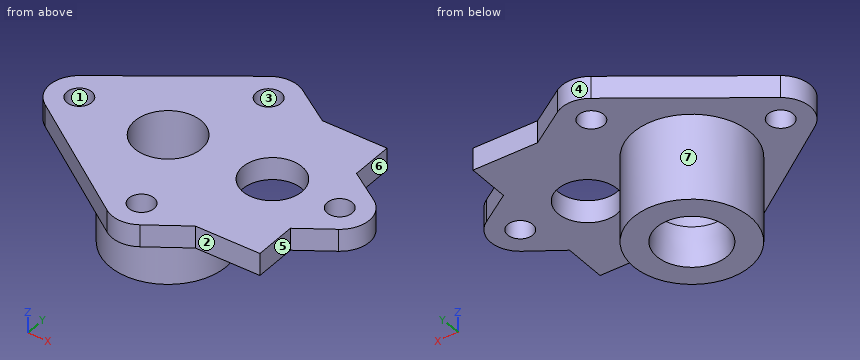
```python
from build123d import *

# Parameters (mm, degrees)
SZKIC1_R                    = 7.9
SZKIC1_R_2                  = 4.75
DODANIE_WYCI_GNI_CIE1_DEPTH = 11.6
DODANIE_WYCI_GNI_CIE2_START = -0.5
SZKIC2_R                    = 4.75
SZKIC2_R_2                  = 4.5
DODANIE_WYCI_GNI_CIE2_DEPTH = 0.5
SFAZOWANIE1_SIZE            = 11.5
SFAZOWANIE1_SIZE_2          = 0.5
SZKIC4_R                    = 4
SZKIC4_R_2                  = 1.7
SZKIC4_R_3                  = 4.5
DODANIE_WYCI_GNI_CIE4_DEPTH = 3
DODANIE_WYCI_GNI_CIE5_DEPTH = 3


with BuildPart() as part:
    # Szkic1 → Dodanie-wyciągnięcie1 (new body)
    with BuildSketch(Plane.XY):
        Circle(SZKIC1_R)
        Circle(SZKIC1_R_2, mode=Mode.SUBTRACT)
    extrude(amount=DODANIE_WYCI_GNI_CIE1_DEPTH)

    # Szkic2 → Dodanie-wyciągnięcie2 (add)
    with BuildSketch(Plane.XY.offset(11.6).offset(DODANIE_WYCI_GNI_CIE2_START)):
        Circle(SZKIC2_R)
        Circle(SZKIC2_R_2, mode=Mode.SUBTRACT)
    extrude(amount=DODANIE_WYCI_GNI_CIE2_DEPTH)

    # Sfazowanie1
    # the kernel refuses this chamfer: 11.5, 0.5 mm, written as the material it adds along each edge
    with BuildSketch(Plane(origin=(0, 0, 11.1), x_dir=(1, 0, 0), z_dir=(0, -1, 0))) as sfazowanie1_piece_1_section:
        Polygon((4.75, -SFAZOWANIE1_SIZE), (4.75 - SFAZOWANIE1_SIZE_2, 0), (4.75, 0), align=None)
    sfazowanie1_piece_1 = revolve(axis=Axis((0, 0, 11.1), (0, 0, 1)), mode=Mode.PRIVATE)
    sfazowanie1_piece_1 = split(sfazowanie1_piece_1, bisect_by=Plane(origin=(-4.668659179, 0, 0), z_dir=(0, 0, 1)), keep=Keep.TOP, mode=Mode.PRIVATE)
    sfazowanie1_piece_1 = sfazowanie1_piece_1 - Plane(origin=(0, 0, 2.677276297), x_dir=(1, 0, 0), z_dir=(0, 0, -1)) * Cylinder(4.5, 46, mode=Mode.PRIVATE)
    add(sfazowanie1_piece_1)

    # Szkic4 → Dodanie-wyciągnięcie4 (add)
    with BuildSketch(Plane.XY.offset(11.6)):
        with BuildLine():
            Line((2.69326721, 15.267871453), (-14.30673279, 3.267871453))
            ThreePointArc((-14.30673279, 3.267871453), (-16, 0), (-14.30673279, -3.267871453))
            Line((-14.30673279, -3.267871453), (2.69326721, -15.267871453))
            ThreePointArc((2.69326721, -15.267871453), (4.936503941, -15.999496), (7.201834862, -15.339449541))
            Line((7.201834862, -15.339449541), (25.401834862, -3.339449541))
            ThreePointArc((25.401834862, -3.339449541), (27.2, 0), (25.401834862, 3.339449541))
            Line((25.401834862, 3.339449541), (7.201834862, 15.339449541))
            ThreePointArc((7.201834862, 15.339449541), (4.936503941, 15.999496), (2.69326721, 15.267871453))
        make_face()
        with Locations((14.1, 0)):
            Circle(SZKIC4_R, mode=Mode.SUBTRACT)
        with Locations((-12, 0)):
            Circle(SZKIC4_R_2, mode=Mode.SUBTRACT)
        with Locations((5, 12)):
            Circle(SZKIC4_R_2, mode=Mode.SUBTRACT)
        with Locations((5, -12)):
            Circle(SZKIC4_R_2, mode=Mode.SUBTRACT)
        with Locations((23.2, 0)):
            Circle(SZKIC4_R_2, mode=Mode.SUBTRACT)
        Circle(SZKIC4_R_3, mode=Mode.SUBTRACT)
    extrude(amount=DODANIE_WYCI_GNI_CIE4_DEPTH)

    # Szkic5 → Dodanie-wyciągnięcie5 (add)
    with BuildSketch(Plane.XY.offset(14.6)):
        Polygon((21, -12), (21, -6.241758242), (12.266666667, -12), align=None)
        Polygon((21, 12), (12.266666667, 12), (21, 6.241758242), align=None)
    extrude(amount=-DODANIE_WYCI_GNI_CIE5_DEPTH)


solid = part.part
```
Geometry: final body of the model. Coordinates: model frame, mm. Face numbers are marked on the shaded views. A direction names the side the tool comes from. Coordinates: 2 decimals unless noted, no trailing zeros. Write each loop counter-clockwise with the first axis right and the second up, starting at its lowest first coordinate (ties: lowest second). Pieces come first, ordered by that corner, then holes. Notation, with made-up numbers: M -27.5,-13.5 L 27.5,-13.5 A27 ccw 27.5,3.5 Z; hole C 86.5,-23 d5. An arc over 180 degrees is marked long. Answer as CSV lines item,"result". Start each with the question number.
Q1. Cut plane D-D on x = 19. Return the cut outline in (y, z).
Q2. Cut plane A-A on x = 14.1. Return the cut outline in (y, z), then the cut area to 3 significant figures.
Q3. Line query: line 1 (Z direction, x = -2.5, y = -11.5); line 2 (X direction, y = -2, z = 13.5); line 3 (X direction, y = -12.5, z = 12). Output: solid intervals per line, ascending. Write a range as from..to.
Q4. Pin query (flat end, axial travel): P1, Ø0.9, axis at x = 15.5, z = 13.5, coming from the +Y side; P2, Ø1.5, axis at y = -3.5, z = 12, coming from the -X side; P3, Ø2.5, axis at x = 5, y = 12, coming from the -Z side; P4, Ø2.5, axis at y = 9.5, z = 12.5, coming from the +X side. Return the tip coordinate at first contact, or that it passes through.
Q5. Reachability of the marked faces 5, 6 and 7 from +Z, -Z, +X, -X, +Y, -Y: full face, straight path, thin tool, end or side. Return the list, or none.
Q6. Cut plane C-C on z = 10.5. Return the cut outline in (x, y).
Q7. Mould query, pull axis Y, two halves, no side actions, for the marked faces 1, 2, 3 and 4. Classes: released by +Y, released by -Y, zero draft, split by the parting line, or undercut.
Q8. Cut plane B-B on y = 11.5. Return the cut outline in (x, z).
Findings below:
1,outline,"M -12,11.6 L 12,11.6 L 12,14.6 L -12,14.6 Z"
2,outline,"M -12,11.6 L -4,11.6 L -4,14.6 L -12,14.6 Z; M 4,11.6 L 12,11.6 L 12,14.6 L 4,14.6 Z"
2,area,"48.0 mm2"
3,line 1,"z = 11.6..14.6"
3,line 2,"x = -15.46..-4.03, 4.03..10.64, 17.56..26.66"
3,line 3,"x = -1.23..3.38, 6.62..11.51"
4,P1,"stops at y = 12"
4,P2,"stops at x = -14.9"
4,P3,"passes through"
4,P4,"stops at x = 21"
5,face 5,"+Z, -Z, +X, -Y"
5,face 6,"+Z, -Z, +X, +Y"
5,face 7,"-Z"
6,outline,"C 0,0 d15.8; hole C 0,0 d9"
7,face 1,"undercut"
7,face 2,"released by -Y"
7,face 3,"undercut"
7,face 4,"released by +Y"
8,outline,"M -2.64,11.6 L 3.38,11.6 L 3.38,14.6 L -2.64,14.6 Z; M 6.62,11.6 L 21,11.6 L 21,14.6 L 6.62,14.6 Z"
